```python
from build123d import *

# Parameters (mm, degrees)
SKETCH1_W           = 79
SKETCH1_H           = 220
BOSS_EXTRUDE1_DEPTH = 20
SKETCH2_W           = 6
SKETCH2_H           = 6
CUT_EXTRUDE1_DEPTH  = 76
SKETCH3_W           = 5
SKETCH3_H           = 5
CUT_EXTRUDE2_DEPTH  = 189
SKETCH4_W           = 5
SKETCH4_H           = 5
CUT_EXTRUDE3_DEPTH  = 100
SKETCH5_W           = 10
SKETCH5_H           = 25
CUT_EXTRUDE4_DEPTH  = 4
FILLET1_R           = 2
SKETCH6_W           = 11
SKETCH6_H           = 25
CUT_EXTRUDE5_DEPTH  = 4.5
FILLET2_R           = 2
SKETCH7_W           = 14
SKETCH7_H           = 35
CUT_EXTRUDE6_DEPTH  = 4
FILLET3_R           = 2
CHAMFER1_SIZE       = 2


with BuildPart() as part:
    # Sketch1 → Boss-Extrude1 (new body)
    with BuildSketch(Plane.XY):
        with Locations((-21, -169)):
            Rectangle(SKETCH1_W, SKETCH1_H)
    extrude(amount=-BOSS_EXTRUDE1_DEPTH)

    # Sketch2 → Cut-Extrude1 (cut)
    with BuildSketch(Plane(origin=(0, -59, 0), x_dir=(1, 0, 0), z_dir=(0, 1, 0))):
        with Locations((-33.166666667, 18.5)):
            Rectangle(SKETCH2_W, SKETCH2_H)
    extrude(amount=-CUT_EXTRUDE1_DEPTH, mode=Mode.SUBTRACT)

    # Sketch3 → Cut-Extrude2 (cut)
    with BuildSketch(Plane(origin=(0, -59, 0), x_dir=(1, 0, 0), z_dir=(0, 1, 0))):
        with Locations((-21.001666667, 18.5)):
            Rectangle(SKETCH3_W, SKETCH3_H)
    extrude(amount=-CUT_EXTRUDE2_DEPTH, mode=Mode.SUBTRACT)

    # Sketch4 → Cut-Extrude3 (cut)
    with BuildSketch(Plane(origin=(0, -59, 0), x_dir=(1, 0, 0), z_dir=(0, 1, 0))):
        with Locations((-8.835, 18.5)):
            Rectangle(SKETCH4_W, SKETCH4_H)
    extrude(amount=-CUT_EXTRUDE3_DEPTH, mode=Mode.SUBTRACT)

    # Sketch5 → Cut-Extrude4 (cut)
    with BuildSketch(Plane(origin=(0, 0, -20), x_dir=(-1, 0, 0), z_dir=(0, 0, -1))):
        with Locations((8.835, -146.496976588)):
            Rectangle(SKETCH5_W, SKETCH5_H)
    extrude(amount=-CUT_EXTRUDE4_DEPTH, mode=Mode.SUBTRACT)

    # Fillet1
    fillet1_edges = [part.edges().sort_by_distance(p)[0] for p in [
        (-13.835, -158.996976588, -18),
        (-3.835, -133.996976588, -18),
        (-13.835, -133.996976588, -18),
        (-3.835, -158.996976588, -18),
    ]]
    fillet(fillet1_edges, radius=FILLET1_R)

    # Sketch6 → Cut-Extrude5 (cut)
    with BuildSketch(Plane(origin=(0, 0, -20), x_dir=(-1, 0, 0), z_dir=(0, 0, -1))):
        with Locations((33.166666667, -122.5)):
            Rectangle(SKETCH6_W, SKETCH6_H)
    extrude(amount=-CUT_EXTRUDE5_DEPTH, mode=Mode.SUBTRACT)

    # Fillet2
    fillet2_edges = [part.edges().sort_by_distance(p)[0] for p in [
        (-38.666666667, -135, -17.75),
        (-27.666666667, -110, -17.75),
        (-38.666666667, -110, -17.75),
        (-27.666666667, -135, -17.75),
    ]]
    fillet(fillet2_edges, radius=FILLET2_R)

    # Sketch7 → Cut-Extrude6 (cut)
    with BuildSketch(Plane(origin=(0, 0, -20), x_dir=(-1, 0, 0), z_dir=(0, 0, -1))):
        with Locations((21.001666667, -252)):
            Rectangle(SKETCH7_W, SKETCH7_H)
    extrude(amount=-CUT_EXTRUDE6_DEPTH, mode=Mode.SUBTRACT)

    # Fillet3
    fillet3_edges = [part.edges().sort_by_distance(p)[0] for p in [
        (-14.001666667, -234.5, -18),
        (-14.001666667, -269.5, -18),
        (-28.001666667, -269.5, -18),
        (-28.001666667, -234.5, -18),
    ]]
    fillet(fillet3_edges, radius=FILLET3_R)

    # Chamfer1
    chamfer1_edges = [part.edges().sort_by_distance(p)[0] for p in [
        (18.5, -279, -10),
        (-60.5, -279, -10),
        (-60.5, -59, -10),
        (18.5, -59, -10),
    ]]
    chamfer(chamfer1_edges, length=CHAMFER1_SIZE)


solid = part.part
```
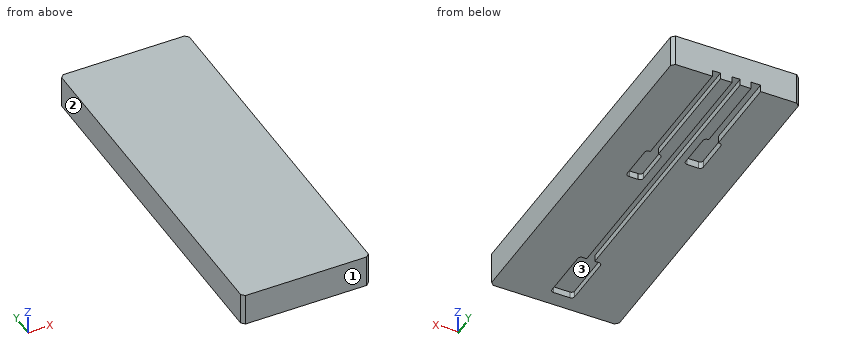
Input: part model. Units: mm. Frame: model coordinates. Face numbers are marked on the shaded views. Give positions to 0.01 mm unless a question says otherwise; leave off trailing zeros. Write each loop counter-clockwise with the first axis right and the second up, starting at its lowest first coordinate (ties: lowest second). Pieces come first, ordered by that corner, then holes. Notation, with made-up numbers: (71, 61.5) - (104, 61.5) arc R11 cw to (104, 72.5) - close; hole circle Ø10 at (64.25, 59.25). An arc over 180 degrees is marked (long way). Write item = value, one per line. Start each with the question number.
1) Cut plane C-C (y = -106.5). Return loops of the section in (x, z) (3 decimals), and give its area (3 significant figures).
2) Cut plane D-D (y = -252.5). Return loops of the section in (x, z), and give its area (3 significant figures).
3) Cut plane B-B (x = -8.5). Return loops of the section in (y, z), and give its area (3 significant figures).
4) Draft query along X for the marked faces 1, 2 and 3. Return one class per face: pulls with the +X half, pulls with the -X half, needs draft (parallel to the pull), parting line crosses it, or undercut.
5) Cut plane A-A (y = -144.5). Return loops of the section in (x, z) (3 decimals).
6) Material intervals for L1, parallel to X at y = -116, z = -17.5 (3 decimals); L2, parallel to Z at x = -20, y = -142.5; L3, parallel to Y at x = -5, z = -18, sorted ascending. Write a range as [from, to].
Answers follow:
q1.outline = (-60.5, -20) - (-36.167, -20) - (-36.167, -15.5) - (-30.167, -15.5) - (-30.167, -20) - (-23.502, -20) - (-23.502, -16) - (-18.502, -16) - (-18.502, -20) - (-11.335, -20) - (-11.335, -16) - (-6.335, -16) - (-6.335, -20) - (18.5, -20) - (18.5, 0) - (-60.5, 0) - close
q1.area = 1,510 mm^2
q2.outline = (-60.5, -20) - (-28, -20) - (-28, -16) - (-14, -16) - (-14, -20) - (18.5, -20) - (18.5, 0) - (-60.5, 0) - close
q2.area = 1,520 mm^2
q3.outline = (-279, -20) - (-159, -20) - (-159, -16) - (-59, -16) - (-59, 0) - (-279, 0) - close
q3.area = 4,000 mm^2
q4.face_1 = needs draft
q4.face_2 = pulls with the -X half
q4.face_3 = undercut
q5.outline = (-60.5, -20) - (-23.502, -20) - (-23.502, -16) - (-18.502, -16) - (-18.502, -20) - (-13.835, -20) - (-13.835, -16) - (-3.835, -16) - (-3.835, -20) - (18.5, -20) - (18.5, 0) - (-60.5, 0) - close
q6.L1 = [-60.5, -38.667], [-27.667, -23.502], [-18.502, -11.335], [-6.335, 18.5]
q6.L2 = [-16, 0]
q6.L3 = [-279, -158.81], [-134.18, -59]
